Verification items for the finished model (mm, model axes). Give positions to 0.01 mm unless a question says otherwise; leave off trailing zeros. Write each loop counter-clockwise with the first axis right and the second up, starting at its lowest first coordinate (ties: lowest second). Pieces come first, ordered by that corner, then holes. Notation, with made-up numbers: (6.25, -33.5) - (33.25, -33.5) arc R20 cw to (33.25, -18.5) - close; hole circle Ø1 at (82, 43). An arc over 180 degrees is marked (long way). Answer as a JSON object with one key per item and string values. Group by question number.
Item 1: Sectioned sample at B-B, the plane x = 226. Record the boundary of the cut face in (y, z).
Item 2: Sectioned sample at A-A, the plane y = 9. Record the boundary of the cut face in (x, z), and give its area (3 significant figures).
Item 3: Sectioned sample at C-C, the plane z = 173.5. Record the boundary of the cut face in (x, y).
Item 4: Scan lines: line 1 along X through (y, z) = (15.5, 577); line 2 along X through (y, z) = (3.25, 326); line 3 along Z through (x, y) = (398.5, 17.25). Record each from-to range of solid material in increasing order. Write a range as [from, to].
Item 5: Go/stop test with a flat-tipped pin: pin 1 (10 mm diameter, centred on x = 369, y = 14.5, fed in from +Z). Record where the tip stops, or that it passes through.
```python
from build123d import *

# Parameters (mm, degrees)
PAD_DEPTH = 19
FILLET_R  = 30


with BuildPart() as part:
    # Sketch001 → Pad (new body)
    with BuildSketch(Plane.XZ):
        Polygon((-39.638222, -29.378442), (-39.638222, 140.621558), (101.719132, 536.468218), (158.152455, 691.5175), (435.361778, 590.621558), (435.361778, -29.378442), align=None)
    extrude(amount=-PAD_DEPTH)

    # Fillet
    fillet_edges = [part.edges().sort_by_distance(p)[0] for p in [
        (-39.638222, 9.5, 140.621558),
        (-39.638222, 9.5, -29.378442),
        (158.152455, 9.5, 691.5175),
        (435.361778, 9.5, 590.621558),
        (435.361778, 9.5, -29.378442),
    ]]
    fillet(fillet_edges, radius=FILLET_R)


solid = part.part
```
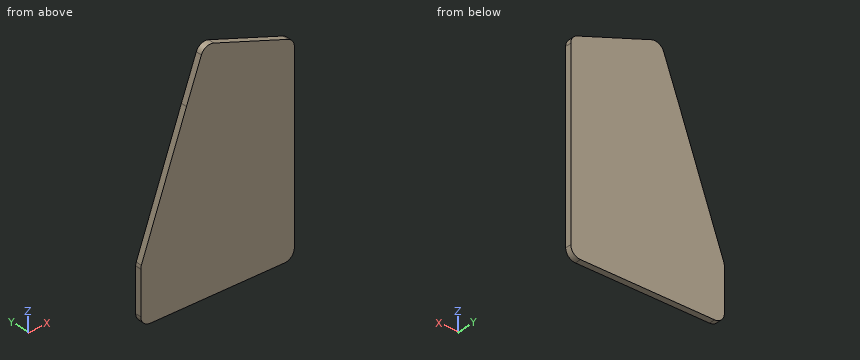
Geometry check:
{
 "1": {"outline": "(0, -29.38) - (19, -29.38) - (19, 666.82) - (0, 666.82) - close"},
 "2": {"outline": "(-39.64, 0.62) arc R30 ccw to (-9.64, -29.38) - (405.36, -29.38) arc R30 ccw to (435.36, 0.62) - (435.36, 569.62) arc R30 ccw to (415.62, 597.81) - (186.34, 681.26) arc R30 ccw to (147.89, 663.33) - (101.72, 536.47) - (-37.89, 145.51) arc R30 ccw to (-39.64, 135.43) - close", "area": "274,000 mm^2"},
 "3": {"outline": "(-27.9, 0) - (435.36, 0) - (435.36, 19) - (-27.9, 19) - close"},
 "4": {"line 1": "[116.47, 434.44]", "line 2": "[26.56, 435.36]", "line 3": "[-29.38, 604.04]"},
 "5": {"pin 1": "z = 616.6"}
}
